Design review of the part built by this model. Coordinates are the model's own, in mm. A direction names the side the tool comes from. Give positions to 0.01 mm unless a question says otherwise; leave off trailing zeros. Order: outer loops, then holes, each group sorted by start corner. A loop starts at its lowest first (then second) coordinate and runs counter-clockwise, first axis right, second up. Notation, with made-up numbers: M 18,38.25 L 49,38.25 A25 cw 49,71.25 Z; hole C -9.75,63 d9. An arc over 180 degrees is marked long. Answer as a JSON object with one key per item and string values.
from build123d import *

# Parameters (mm, degrees)
F0_W     = 28.575
F0_H     = 10.16
F1_DEPTH = 12.192
F2_W     = 28.575
F2_H     = 2.794
F3_DEPTH = 10.9728
F4_R     = 1.905
F5_DEPTH = 25.4


with BuildPart() as f1:
    # F0 (on Top) → F1 (new body)
    with BuildSketch(Plane.XY):
        Rectangle(F0_W, F0_H)
    extrude(amount=F1_DEPTH)

    # F2 (on face) → F3 (cut)
    with BuildSketch(Plane.XY.offset(12.192)):
        Rectangle(F2_W, F2_H)
    extrude(amount=-F3_DEPTH, mode=Mode.SUBTRACT)

    # F4 (on face) → F5 (cut)
    with BuildSketch(Plane.XZ.offset(5.08)):
        with Locations((-8.50641, 6.096)):
            Circle(F4_R)
        with Locations((7.61332, 6.096)):
            Circle(F4_R)
    extrude(amount=-F5_DEPTH, mode=Mode.SUBTRACT)


solid = f1.part
(1) We need section C-C (x = -3.5). Write out the cut boundary in (y, z).
Checked values:
{"outline": "M -5.08,0 L 5.08,0 L 5.08,12.19 L 1.4,12.19 L 1.4,1.22 L -1.4,1.22 L -1.4,12.19 L -5.08,12.19 Z"}
(2) To check wall thickness, follow L1, parallel to Y at x = -13, z = 2.5; L2, parallel to X at y = 1.5, z = 7; L3, parallel to X at y = 2, z = 6.75. State the ranges of each line that lie inside material, in increasing order. Write a range as from..to.
Checked values:
{"L1": "y = -5.08..-1.4, 1.4..5.08", "L2": "x = -14.29..-10.18, -6.83..5.94, 9.29..14.29", "L3": "x = -14.29..-10.3, -6.72..5.82, 9.4..14.29"}
(3) We need section B-B (x = 6). Write out the cut boundary in (y, z), plus the area to 3 significant figures.
Checked values:
{"outline": "M -5.08,0 L 5.08,0 L 5.08,5.08 L 1.4,5.08 L 1.4,1.22 L -1.4,1.22 L -1.4,5.08 L -5.08,5.08 Z; M -5.08,7.11 L -1.4,7.11 L -1.4,12.19 L -5.08,12.19 Z; M 1.4,7.11 L 5.08,7.11 L 5.08,12.19 L 1.4,12.19 Z", "area": "78.3 mm^2"}
(4) We need section A-A (z = 8.75). Write out the cut boundary in (x, y).
Checked values:
{"outline": "M -14.29,-5.08 L 14.29,-5.08 L 14.29,-1.4 L -14.29,-1.4 Z; M -14.29,1.4 L 14.29,1.4 L 14.29,5.08 L -14.29,5.08 Z"}
(5) Draft analysis for pull direction X (two halves, no side actions). For faces 1 (the flat face through (-14.288, -2, 6)), 2 (the flat face through (0, 3, 12.192)), 3 (the cylindrical face through (7.365, -3.264, 7.985)), state which applies: +X half, -X half, draft (parallel to the pull), parting line (faces both ways), or undercut.
Checked values:
{"face 1": "-X half", "face 2": "draft", "face 3": "undercut"}
(6) We need section D-D (z = 7.25). Write out the cut boundary in (x, y).
Checked values:
{"outline": "M -14.29,-5.08 L -10.02,-5.08 L -10.02,-1.4 L -14.29,-1.4 Z; M -14.29,1.4 L -10.02,1.4 L -10.02,5.08 L -14.29,5.08 Z; M -6.99,-5.08 L 6.1,-5.08 L 6.1,-1.4 L -6.99,-1.4 Z; M -6.99,1.4 L 6.1,1.4 L 6.1,5.08 L -6.99,5.08 Z; M 9.13,-5.08 L 14.29,-5.08 L 14.29,-1.4 L 9.13,-1.4 Z; M 9.13,1.4 L 14.29,1.4 L 14.29,5.08 L 9.13,5.08 Z"}
(7) Tool access review of faces 4 (the flat face through (0, 5.08, 6)), 5 (the flat face through (0, 1.397, 7)): name each direction out of +Z, -Z, +X, -X, +Y, -Y from which nothing blocks a thin tool from reaching the whole face with its end or side.
Checked values:
{"face 4": "+Z, -Z, +X, -X, +Y", "face 5": "+Z, +X, -X"}
